Work out the finished part from the listing and answer in its coordinate system (mm). A direction names the side the tool comes from. Round coordinates to 2 decimals unless told otherwise and drop trailing zeros. Order: outer loops, then holes, each group sorted by start corner. A loop starts at its lowest first (then second) coordinate and runs counter-clockwise, first axis right, second up. Notation, with made-up numbers: (32.25, 3) -> (47.25, 3) arc R33 cw to (47.25, 32) -> close; hole circle Ø7 at (-8, 69). An arc over 180 degrees is marked (long way). Use a Markdown table: item, result. Add a question column.
Item 1: For a pull along X with two mould halves and no side action, classify faces 1 (the flat face through (-280, -210, -533)), 2 (the flat face through (260, 230, -533)) as +X half, -X half, draft (parallel to the pull), parting line (faces both ways), or undercut.
Item 2: Find the intervals of material crossed by L1, parallel to Y at x = 320, z = -1075.25; L2, parallel to Y at x = -286, z = -687; L3, parallel to Z at x = -282, y = -202, in increasing order. Write a range as [from, to].
Item 3: Flat-ended cylindrical pins translate along their axes: P1, Ø12, axis at x = -277.5, y = -59, coming from the +Z side; P2, Ø20, axis at x = -326.5, y = -213.5, coming from the +Z side; P3, Ø20, axis at y = 103, z = -1063, coming from the +X side. Find the tip coordinate at first contact, or state that the pin passes through.
Item 4: A cutting plane is placed at D-D, the plane y = -56. Determine the outline of the cut face in (x, z), plus the area to 3 significant figures.
Item 5: A cutting plane is placed at A-A, the plane y = -185. Determine the outline of the cut face in (x, z).
Item 6: A cutting plane is placed at C-C, the plane x = -21. Determine the outline of the cut face in (y, z), plus the area to 3 significant figures.
Item 7: A cutting plane is placed at B-B, the plane z = -482.5. Determine the outline of the cut face in (x, y), plus the area to 3 significant figures.
Item 8: A tool of negligible diameter and unlimited length cuts with its end or side. For faces 3 (the flat face through (-260, 3, -1060)), 4 (the flat face through (-325, 201, -1070)), 5 (the flat face through (-4, -230, -1040)), 6 (the flat face through (280, -210, -533)), from which of +Z, -Z, +X, -X, +Y, -Y can it reach the whole face along a straight path? Write none if from no direction.
from build123d import *

# Parameters (mm, degrees)
F0_W     = 40
F0_H     = 500
F1_DEPTH = 40
F2_W     = 40
F2_H     = 40
F3_DEPTH = 1000
F4_W     = 600
F4_H     = 500
F4_W_2   = 520
F4_H_2   = 420
F5_DEPTH = 40
F6_W     = 40
F6_H     = 80
F6_R     = 10
F7_DEPTH = 10
F8_W     = 600
F8_H     = 500
F9_DEPTH = 40


with BuildPart() as f1:
    # F0 (on Top) → F1 (new body)
    with BuildSketch(Plane.XY):
        with Locations((280, 0)):
            Rectangle(F0_W, F0_H)
        with Locations((-280, 0)):
            Rectangle(F0_W, F0_H)
    extrude(amount=-F1_DEPTH)

    # F2 (on face) → F3 (join)
    with BuildSketch(Plane(origin=(0, 0, -40), x_dir=(1, 0, 0), z_dir=(0, 0, -1))):
        with Locations((280, -230)):
            Rectangle(F2_W, F2_H)
        with Locations((-280, -230)):
            Rectangle(F2_W, F2_H)
        with Locations((280, 230)):
            Rectangle(F2_W, F2_H)
        with Locations((-280, 230)):
            Rectangle(F2_W, F2_H)
    extrude(amount=F3_DEPTH)

    # F4 (on face) → F5 (join)
    with BuildSketch(Plane(origin=(0, 0, -1040), x_dir=(1, 0, 0), z_dir=(0, 0, -1))):
        Rectangle(F4_W, F4_H)
        Rectangle(F4_W_2, F4_H_2, mode=Mode.SUBTRACT)
    extrude(amount=F5_DEPTH)

    # F6 (on face) → F7 (join)
    with BuildSketch(Plane(origin=(0, 0, -1080), x_dir=(1, 0, 0), z_dir=(0, 0, -1))):
        with Locations((-320, 210)):
            Rectangle(F6_W, F6_H)
        with Locations((-320, 210)):
            Circle(F6_R, mode=Mode.SUBTRACT)
        with Locations((320, 210)):
            Rectangle(F6_W, F6_H)
        with Locations((320, 210)):
            Circle(F6_R, mode=Mode.SUBTRACT)
        with Locations((-320, -210)):
            Rectangle(F6_W, F6_H)
        with Locations((-320, -210)):
            Circle(F6_R, mode=Mode.SUBTRACT)
        with Locations((320, -210)):
            Rectangle(F6_W, F6_H)
        with Locations((320, -210)):
            Circle(F6_R, mode=Mode.SUBTRACT)
    extrude(amount=-F7_DEPTH)

    # F8 (on face) → F9 (cut)
    with BuildSketch(Plane.XY):
        Rectangle(F8_W, F8_H)
    extrude(amount=-F9_DEPTH, mode=Mode.SUBTRACT)


solid = f1.part
Reported:
| question | item | result |
|---|---|---|
| 1 | face 1 | draft |
| 1 | face 2 | undercut |
| 2 | L1 | [-250, -220], [-200, -170], [170, 200], [220, 250] |
| 2 | L2 | [-250, -210], [210, 250] |
| 2 | L3 | [-1080, -1040] |
| 3 | P1 | z = -1040 |
| 3 | P2 | z = -1070 |
| 3 | P3 | x = 300 |
| 4 | outline | (-300, -1080) -> (-260, -1080) -> (-260, -1040) -> (-300, -1040) -> close; (260, -1080) -> (300, -1080) -> (300, -1040) -> (260, -1040) -> close |
| 4 | area | 3,200 mm² |
| 5 | outline | (-340, -1080) -> (-260, -1080) -> (-260, -1040) -> (-300, -1040) -> (-300, -1070) -> (-340, -1070) -> close; (260, -1080) -> (340, -1080) -> (340, -1070) -> (300, -1070) -> (300, -1040) -> (260, -1040) -> close |
| 6 | outline | (-250, -1080) -> (-210, -1080) -> (-210, -1040) -> (-250, -1040) -> close; (210, -1080) -> (250, -1080) -> (250, -1040) -> (210, -1040) -> close |
| 6 | area | 3,200 mm² |
| 7 | outline | (-300, -250) -> (-260, -250) -> (-260, -210) -> (-300, -210) -> close; (-300, 210) -> (-260, 210) -> (-260, 250) -> (-300, 250) -> close; (260, -250) -> (300, -250) -> (300, -210) -> (260, -210) -> close; (260, 210) -> (300, 210) -> (300, 250) -> (260, 250) -> close |
| 7 | area | 6,400 mm² |
| 8 | face 3 | +Z, -Z |
| 8 | face 4 | +Z, -X, +Y, -Y |
| 8 | face 5 | +Z, +Y, -Y |
| 8 | face 6 | +Z, +X, -X |
